Build history of the part. All positions in model axes, mm. Coordinates: 2 decimals unless noted, no trailing zeros. Write each loop counter-clockwise with the first axis right and the second up, starting at its lowest first coordinate (ties: lowest second). Pieces come first, ordered by that corner, then holes. Notation, with made-up numbers: (-37, 58.5) -> (-11, 58.5) arc R24 ccw to (-11, 95.5) -> close; hole circle Ø10 at (33, 41). An arc over 180 degrees is marked (long way). Write each question's results on one line, items separated by ' | '. Start each with the question number.
Q1. Drop flat-ended pins along their axis: pin 1 Ø4 at (x, z) = (7.5, 0) entering from -Y; pin 2 Ø1 at (x, y) = (5, 2) entering from -Z. Give the stop position or say it passes through.
Q2. Saw through at D-D on y = 0.4. Give the cut face in (x, z).
Q3. Saw through at A-A on z = 0. Give the cut face in (x, y), and give its area (3 significant figures).
Q4. Two-plate mould, pull along Z, no slides. Class faces 1 (the face through (5, 0, 2)), 2 (the face through (-0.27, 2.46, -6.28)), 3 (the face through (-9.76, 2.46, -2.17)): released by +Z, released by -Z, zero draft, split by the parting line, or undercut.
Q5. Saw through at B-B on x = 0. Give the cut face in (y, z).
Q6. Saw through at C-C on x = 4.5. Give the cut face in (y, z), and give its area (3 significant figures).
Q7. Drill centre lines: line 1 (X direction, y = 2.1, z = 0); line 2 (Z direction, x = -0.5, y = 0.85). Where is each one in solid material? Low to high.
from build123d import *

# Parameters (mm, degrees)
SKETCH1_R             = 10
BOSS_EXTRUDE1_DEPTH   = 5
SKETCH2_R             = 5
CUT_EXTRUDE1_DEPTH    = 16
SKETCH3_R             = 1.25
CUT_EXTRUDE2_DEPTH    = 5
CIRPATTERN1_OUTLINE_R = 1.25
CIRPATTERN1_DEPTH     = 5


# Read off the part's stored shape, not the designer's step: CirPattern1
with BuildPart() as part:
    # Sketch1 → Boss-Extrude1 (new body)
    with BuildSketch(Plane(origin=(0, 0, 0), x_dir=(1, 0, 0), z_dir=(0, 1, 0))):
        with Locations(Location((0, 0, 0), (0, 0, 270))):
            Circle(SKETCH1_R)
    extrude(amount=BOSS_EXTRUDE1_DEPTH)

    # Sketch2 → Cut-Extrude1 (cut, through all)
    with BuildSketch(Plane(origin=(0, 0, 0), x_dir=(1, 0, 0), z_dir=(0, 1, 0))):
        with Locations(Location((0, 0, 0), (0, 0, 270))):
            Circle(SKETCH2_R)
    extrude(amount=CUT_EXTRUDE1_DEPTH, mode=Mode.SUBTRACT)

    # Sketch3 → Cut-Extrude2 (cut)
    with BuildSketch(Plane(origin=(0, 5, 0), x_dir=(1, 0, 0), z_dir=(0, 1, 0))):
        with Locations(Location((-7.5, 0, 0), (0, 0, 270))):
            Circle(SKETCH3_R)
    extrude(amount=-CUT_EXTRUDE2_DEPTH, mode=Mode.SUBTRACT)

    # CirPattern1 outline → CirPattern1 (cut)
    with BuildSketch(Plane(origin=(0, 0, 0), x_dir=(1, 0, 0), z_dir=(0, 1, 0))):
        with Locations((0, 7.5)):
            Circle(CIRPATTERN1_OUTLINE_R)
        with Locations((7.5, 0)):
            Circle(CIRPATTERN1_OUTLINE_R)
        with Locations((0, -7.5)):
            Circle(CIRPATTERN1_OUTLINE_R)
    extrude(amount=CIRPATTERN1_DEPTH, mode=Mode.SUBTRACT)


solid = part.part
Returned:
1) pin 1: stops at y = 0 | pin 2: stops at z = -8.93
2) outline: circle Ø20 at (0, 0); hole circle Ø2.5 at (-7.5, 0); hole circle Ø10 at (0, 0); hole circle Ø2.5 at (0, -7.5); hole circle Ø2.5 at (0, 7.5); hole circle Ø2.5 at (7.5, 0)
3) outline: (-10, 0) -> (-8.75, 0) -> (-8.75, 5) -> (-10, 5) -> close; (-6.25, 0) -> (-5, 0) -> (-5, 5) -> (-6.25, 5) -> close; (5, 0) -> (6.25, 0) -> (6.25, 5) -> (5, 5) -> close; (8.75, 0) -> (10, 0) -> (10, 5) -> (8.75, 5) -> close | area: 25.0 mm2
4) face 1: zero draft | face 2: undercut | face 3: split by the parting line
5) outline: (0, -10) -> (5, -10) -> (5, -8.75) -> (0, -8.75) -> close; (0, -6.25) -> (5, -6.25) -> (5, -5) -> (0, -5) -> close; (0, 5) -> (5, 5) -> (5, 6.25) -> (0, 6.25) -> close; (0, 8.75) -> (5, 8.75) -> (5, 10) -> (0, 10) -> close
6) outline: (0, -8.93) -> (5, -8.93) -> (5, -2.18) -> (0, -2.18) -> close; (0, 2.18) -> (5, 2.18) -> (5, 8.93) -> (0, 8.93) -> close | area: 67.5 mm2
7) line 1: x = -10 to -8.75, -6.25 to -5, 5 to 6.25, 8.75 to 10 | line 2: z = -9.99 to -8.65, -6.35 to -4.97, 4.97 to 6.35, 8.65 to 9.99
